```python
from build123d import *

# Parameters (mm, degrees)
SKETCH_1_R      = 1.5
EXTRUDE_1_DEPTH = 1.5


with BuildPart() as part:
    # 草图1 → 凸台-拉伸1 (new body)
    with BuildSketch(Plane(origin=(0, 0, 0), x_dir=(1, 0, 0), z_dir=(0, 1, 0))):
        with BuildLine():
            Line((-1, 0), (-18.069602783, 0))
            ThreePointArc((-18.069602783, 0), (-18.776709565, -0.292893219), (-19.069602783, -1))
            Line((-19.069602783, -1), (-19.069602783, -3))
            ThreePointArc((-19.069602783, -3), (-22.069602783, -6), (-25.069602783, -3))
            Line((-25.069602783, -3), (-25.069602783, -1))
            ThreePointArc((-25.069602783, -1), (-25.362496002, -0.292893219), (-26.069602783, 0))
            Line((-26.069602783, 0), (-43, 0))
            ThreePointArc((-43, 0), (-43.707106781, 0.292893219), (-44, 1))
            Line((-44, 1), (-44, 43))
            ThreePointArc((-44, 43), (-43.707106781, 43.707106781), (-43, 44))
            Line((-43, 44), (-26.069602783, 44))
            ThreePointArc((-26.069602783, 44), (-25.362496002, 44.292893219), (-25.069602783, 45))
            Line((-25.069602783, 45), (-25.069602783, 47))
            ThreePointArc((-25.069602783, 47), (-22.069602783, 50), (-19.069602783, 47))
            Line((-19.069602783, 47), (-19.069602783, 45))
            ThreePointArc((-19.069602783, 45), (-18.776709565, 44.292893219), (-18.069602783, 44))
            Line((-18.069602783, 44), (-1, 44))
            ThreePointArc((-1, 44), (-0.292893219, 43.707106781), (0, 43))
            Line((0, 43), (0, 1))
            ThreePointArc((0, 1), (-0.292893219, 0.292893219), (-1, 0))
        make_face()
        with Locations((-22.069602783, -3)):
            Circle(SKETCH_1_R, mode=Mode.SUBTRACT)
        with Locations((-22.069602783, 47)):
            Circle(SKETCH_1_R, mode=Mode.SUBTRACT)
        Polygon((-19.869912149, 24.021868684), (-19.869912149, 22.52053711), (-25.144061861, 18.620495369), (-25.144061861, 20.121826943), align=None, mode=Mode.SUBTRACT)
        Polygon((-20.026597006, 26.682534422), (-20.026597006, 25.181202847), (-22.444035318, 23.393595206), (-22.444035318, 24.894926781), align=None, mode=Mode.SUBTRACT)
        Polygon((-22.65940243, 19.377411479), (-22.65940243, 17.876079904), (-25.076840742, 16.088472263), (-25.076840742, 17.589803838), align=None, mode=Mode.SUBTRACT)
    extrude(amount=EXTRUDE_1_DEPTH)


solid = part.part
```
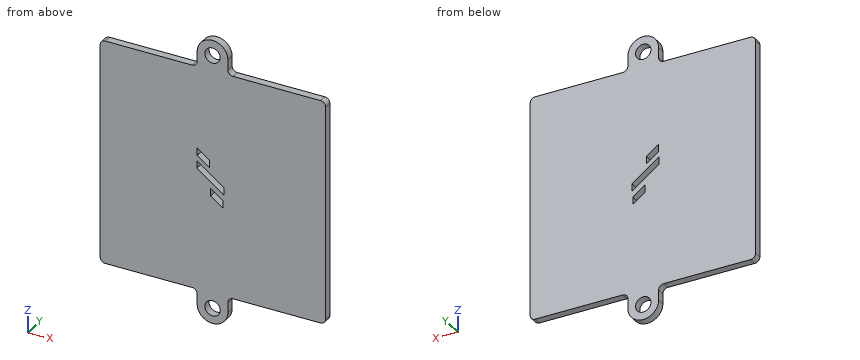
Check sheet for the modelled part. Datum: model origin and axes. Units: mm. Give positions to 0.01 mm unless a question says otherwise; leave off trailing zeros. Order: outer loops, then holes, each group sorted by start corner. A loop starts at its lowest first (then second) coordinate and runs counter-clockwise, first axis right, second up. Notation, with made-up numbers: M 12.5,-16.75 L 17.5,-16.75 A14 cw 17.5,1.25 Z; hole C 31,-20 d3. An arc over 180 degrees is marked long. Answer in a Markdown table with one row per item. Add a question column.
Q1. Sectioned sample at B-B, the plane x = -7. Record the boundary of the cut face in (y, z).
Q2. Thickness scan on L1, parallel to X at y = 1.2, z = -47; L2, parallel to Z at x = -11.5, y = 0.7; L3, parallel to X at y = 1.2, z = -19. Record the ranges inside material, lowest first.
Q3. Sectioned sample at A-A, the plane y = 0.25. Count the separate pieces of the cut face and the enclosed holes in it, and give its area (3 significant figures).
Verdict:
| question | item | result |
|---|---|---|
| 1 | outline | M 0,-44 L 1.5,-44 L 1.5,0 L 0,0 Z |
| 2 | L1 | -25.07 to -23.57, -20.57 to -19.07 |
| 2 | L2 | -44 to 0 |
| 2 | L3 | -44 to -25.14, -24.63 to -23.17, -22.66 to 0 |
| 3 | separate pieces | 1 |
| 3 | enclosed holes | 5 |
| 3 | area | 1,970 mm² |
